from build123d import *

# Parameters (mm, degrees)
F0_R     = 2.5
F0_R_2   = 5
F1_DEPTH = 2
F2_R     = 0.5
F3_SIZE  = 0.5


with BuildPart() as f1:
    # F0 (on Front) → F1 (new body)
    with BuildSketch(Plane.XZ):
        with BuildLine():
            Line((10.978817, 8.515241), (-32.021183, 8.515241))
            ThreePointArc((-32.021183, 8.515241), (-39.521183, 1.015241), (-32.021183, -6.484759))
            Line((-32.021183, -6.484759), (10.978817, -6.484759))
            ThreePointArc((10.978817, -6.484759), (18.478817, 1.015241), (10.978817, 8.515241))
        make_face()
        with Locations((-32.021183, 1.015241)):
            Circle(F0_R, mode=Mode.SUBTRACT)
        with Locations((10.978817, 1.015241)):
            Circle(F0_R_2, mode=Mode.SUBTRACT)
    extrude(amount=F1_DEPTH)

    # F2
    f2_edges = [f1.edges().sort_by_distance(p)[0] for p in [
        (-10.521183, -2, 8.515241),
        (-39.521183, 0, 1.015241),
    ]]
    fillet(f2_edges, radius=F2_R)

    # F3
    f3_edges = [f1.edges().sort_by_distance(p)[0] for p in [
        (-34.521183, -2, 1.015241),
        (5.978817, -2, 1.015241),
        (-34.521183, 0, 1.015241),
        (5.978817, 0, 1.015241),
    ]]
    chamfer(f3_edges, length=F3_SIZE)


solid = f1.part
Check sheet for the modelled part. Datum: model origin and axes. Units: mm. Give positions to 0.01 mm unless a question says otherwise; leave off trailing zeros. Write each loop counter-clockwise with the first axis right and the second up, starting at its lowest first coordinate (ties: lowest second). Pieces come first, ordered by that corner, then holes. Notation, with made-up numbers: (-29, -27) -> (14, -27) arc R12 cw to (14, -18) -> close; hole circle Ø11 at (-19.75, 2.25). An arc over 180 degrees is marked (long way). Write item = value, one per line.
Item 1: Sectioned sample at A-A on y = -1. Record the boundary of the cut face in (x, z), and give its area (3 significant figures).
Output:
outline = (-32.02, -6.48) -> (10.98, -6.48) arc R7.5 ccw to (10.98, 8.52) -> (-32.02, 8.52) arc R7.5 ccw to start; hole circle Ø5 at (-32.02, 1.02); hole circle Ø10 at (10.98, 1.02)
area = 724 mm^2
Item 2: Sectioned sample at B-B on z = -1. Count the separate pieces of the cut face and the enclosed holes in it, and give its area (3 significant figures).
Output:
separate_pieces = 3
enclosed_holes = 0
area = 89.1 mm^2
Item 3: Gauge pin test, flat end, axial feed: pin 1 (4 mm diameter, centred on x = -32.02, z = 1.02, fed in from -Y). Record the tip position at first contact, or that the pin passes through.
Output:
pin_1 = through
Item 4: Scan lines: probe 1 along Z at (x, y) = (-14, -1.55); probe 2 along X at (y, z) = (-0.35, -2); probe 3 along X at (y, z) = (-1.85, 5.75). Record each from-to range of solid material in increasing order. Write a range as from..to.
Output:
probe_1 = -6.48..8.51
probe_2 = -38.86..6.8, 15.15..17.82
probe_3 = -37.65..8.49, 13.47..16.61
Item 5: Release check for a two-part mould opening along Z. For faces 1 (the flat face through (-11, -2, 1)), 2 (the cylindrical face through (18.477, -0.993, 0.85)), 3 (the cylindrical face through (5.984, -0.993, 1.235)) record: +Z half, -Z half, draft (parallel to the pull), parting line (faces both ways), or undercut.
Output:
face_1 = draft
face_2 = parting line
face_3 = undercut
